Geometry check sheet. Reference: the model listing, model coordinates, mm. A direction names the side the tool comes from. Round coordinates to 2 decimals unless told otherwise and drop trailing zeros. Write each loop counter-clockwise with the first axis right and the second up, starting at its lowest first coordinate (ties: lowest second). Pieces come first, ordered by that corner, then holes. Notation, with made-up numbers: (9, 66.5) - (30, 66.5) arc R19 ccw to (30, 79.5) - close; hole circle Ø11 at (-27, 18.5). An arc over 180 degrees is marked (long way). Return JSON: item names as keys, results as strings.
```python
from build123d import *

# Parameters (mm, degrees)
SKETCH1_W           = 10
SKETCH1_H           = 10
SKETCH1_R           = 1.25
BOSS_EXTRUDE1_DEPTH = 2
SKETCH2_W           = 5
SKETCH2_H           = 3
BOSS_EXTRUDE2_DEPTH = 2
SKETCH3_W           = 10
SKETCH3_H           = 8.75
BOSS_EXTRUDE3_DEPTH = 2


with BuildPart() as part:
    # Sketch1 → Boss-Extrude1 (new, symmetric)
    with BuildSketch(Plane(origin=(0, 0, 0), x_dir=(1, 0, 0), z_dir=(0, 1, 0))):
        Rectangle(SKETCH1_W, SKETCH1_H)
        with Locations(Location((0, 0, 0), (0, 0, 270))):
            Circle(SKETCH1_R, mode=Mode.SUBTRACT)
    extrude(amount=BOSS_EXTRUDE1_DEPTH, both=True)

    # Sketch2 → Boss-Extrude2 (add, symmetric)
    with BuildSketch(Plane(origin=(0, 0, 0), x_dir=(1, 0, 0), z_dir=(0, 1, 0))):
        with Locations((0, 6.5)):
            Rectangle(SKETCH2_W, SKETCH2_H)
    extrude(amount=BOSS_EXTRUDE2_DEPTH, both=True)

    # Sketch3 → Boss-Extrude3 (add, symmetric)
    with BuildSketch(Plane(origin=(0, 0, 0), x_dir=(1, 0, 0), z_dir=(0, 1, 0))):
        with Locations((0, 12.375)):
            Rectangle(SKETCH3_W, SKETCH3_H)
    extrude(amount=BOSS_EXTRUDE3_DEPTH, both=True)


solid = part.part
```
(1) Release check for a two-part mould opening along Z. For faces 4 (the face through (-5, 0, 0)), 5 (the face through (0, 0, 5)), 6 (the face through (-2.5, 0, -6)), 7 (the face through (-4, 0, -5)) record: pulls with the +Z half, pulls with the -Z half, needs draft (parallel to the pull), parting line crosses it, or undercut.
Response values:
{"face 4": "needs draft", "face 5": "pulls with the +Z half", "face 6": "undercut", "face 7": "undercut"}
(2) Access from +Z, -Z, +X, -X, +Y, -Y to the whole of each face (thin tool, end or side, straight path). Record for faces 1 (the face through (-1.22, -0.03, -0.27)), 2 (the face through (-4, 0, -8)), 3 (the face through (2.5, 0, -6)).
Response values:
{"face 1": "+Y, -Y", "face 2": "-X, +Y, -Y", "face 3": "+X, +Y, -Y"}
(3) Gauge pin test, flat ends, axial feed: pin 1 (3 mm diameter, centred on x = 0, z = 0, fed in from -Y); pin 2 (1.5 mm diameter, centred on y = 0.5, z = -6.5, fed in from +X). Record the tip position at first contact, or that the pin passes through.
Response values:
{"pin 1": "stops at y = -2", "pin 2": "stops at x = 2.5"}
(4) Material ranges on line 1 along Z through (x, y) = (4, 1.05); line 2 along X through (y, z) = (-0.5, 0); line 3 along X through (y, z) = (1.6, -7.75), recorded low to high. Write a range as [from, to].
Response values:
{"line 1": "z = [-16.75, -8], [-5, 5]", "line 2": "x = [-5, -1.25], [1.25, 5]", "line 3": "x = [-2.5, 2.5]"}
(5) Section check D-D, the plane z = -7. Enter the section's corners in (x, y).
Response values:
{"outline": "(-2.5, -2) - (2.5, -2) - (2.5, 2) - (-2.5, 2) - close"}
(6) Section check B-B, the plane x = 0. Enter the section's corners in (y, z).
Response values:
{"outline": "(-2, -16.75) - (2, -16.75) - (2, -1.25) - (-2, -1.25) - close; (-2, 1.25) - (2, 1.25) - (2, 5) - (-2, 5) - close"}
(7) Section check C-C, the plane y = 1.3. Enter the section's corners in (x, z), plus the area to 3 significant figures.
Response values:
{"outline": "(-5, -16.75) - (5, -16.75) - (5, -8) - (2.5, -8) - (2.5, -5) - (5, -5) - (5, 5) - (-5, 5) - (-5, -5) - (-2.5, -5) - (-2.5, -8) - (-5, -8) - close; hole circle Ø2.5 at (0, 0)", "area": "198 mm^2"}
(8) Section check A-A, the plane z = 0. Enter the section's corners in (x, y), plus the area to 3 significant figures.
Response values:
{"outline": "(-5, -2) - (-1.25, -2) - (-1.25, 2) - (-5, 2) - close; (1.25, -2) - (5, -2) - (5, 2) - (1.25, 2) - close", "area": "30.0 mm^2"}
